```python
from build123d import *

# Parameters (mm, degrees)
SKETCH_1_R          = 70
EXTRUDE_1_DEPTH     = 525
SKETCH_2_OUTSIDE_W  = 254.218
SKETCH_2_OUTSIDE_H  = 254.218
SKETCH_2_OUTSIDE_R  = 45
CUT_EXTRUDE_2_DEPTH = 285
CUT_EXTRUDE_START   = -20
SKETCH_3_OUTSIDE_W  = 254.218
SKETCH_3_OUTSIDE_H  = 254.218
SKETCH_3_OUTSIDE_R  = 60
CUT_EXTRUDE_3_DEPTH = 282.703496831
SKETCH_4_OUTSIDE_W  = 254.218
SKETCH_4_OUTSIDE_H  = 254.218
SKETCH_4_OUTSIDE_R  = 37.5
CUT_EXTRUDE_4_DEPTH = 232.5
SKETCH_5_OUTSIDE_W  = 254.218
SKETCH_5_OUTSIDE_H  = 254.218
SKETCH_5_OUTSIDE_R  = 37.5
CUT_EXTRUDE_5_DEPTH = 120
CUT_EXTRUDE_START_2 = 50
CUT_EXTRUDE_6_DEPTH = 485.251813287
SKETCH_8_OUTSIDE_W  = 254.218
SKETCH_8_OUTSIDE_H  = 254.218
SKETCH_8_OUTSIDE_R  = 34
CUT_EXTRUDE_1_DEPTH = 130
CUT_EXTRUDE_START_3 = 30.5
CUT_EXTRUDE_7_DEPTH = 504.751813287
FILLET_1_R          = 5


with BuildPart() as part:
    # 草图1 → 拉伸1 (new body)
    with BuildSketch(Plane(origin=(0, 0, 0), x_dir=(0, 0, -1), z_dir=(1, 0, 0))):
        Circle(SKETCH_1_R)
    extrude(amount=EXTRUDE_1_DEPTH)

    # 草图2 outside → 拉伸2 (cut)
    with BuildSketch(Plane(origin=(525, 0, 0), x_dir=(0, 0, -1), z_dir=(1, 0, 0))):
        Rectangle(SKETCH_2_OUTSIDE_W, SKETCH_2_OUTSIDE_H)
        Circle(SKETCH_2_OUTSIDE_R, mode=Mode.SUBTRACT)
    extrude(amount=-CUT_EXTRUDE_2_DEPTH, mode=Mode.SUBTRACT)

    # 草图3 outside → 拉伸3 (cut, through all)
    with BuildSketch(Plane(origin=(240, 0, 0), x_dir=(0, 0, -1), z_dir=(1, 0, 0)).offset(CUT_EXTRUDE_START)):
        Rectangle(SKETCH_3_OUTSIDE_W, SKETCH_3_OUTSIDE_H)
        Circle(SKETCH_3_OUTSIDE_R, mode=Mode.SUBTRACT)
    extrude(amount=-CUT_EXTRUDE_3_DEPTH, mode=Mode.SUBTRACT)

    # 草图4 outside → 拉伸4 (cut)
    with BuildSketch(Plane(origin=(525, 0, 0), x_dir=(0, 0, -1), z_dir=(1, 0, 0))):
        Rectangle(SKETCH_4_OUTSIDE_W, SKETCH_4_OUTSIDE_H)
        Circle(SKETCH_4_OUTSIDE_R, mode=Mode.SUBTRACT)
    extrude(amount=-CUT_EXTRUDE_4_DEPTH, mode=Mode.SUBTRACT)

    # 草图5 outside → 拉伸5 (cut)
    with BuildSketch(Plane.ZY):
        Rectangle(SKETCH_5_OUTSIDE_W, SKETCH_5_OUTSIDE_H)
        with Locations(Location((0, 0, 0), (0, 0, 180))):
            Circle(SKETCH_5_OUTSIDE_R, mode=Mode.SUBTRACT)
    extrude(amount=-CUT_EXTRUDE_5_DEPTH, mode=Mode.SUBTRACT)

    # 草图6 → 拉伸6 (cut, through all)
    with BuildSketch(Plane.XY.offset(CUT_EXTRUDE_START_2)):
        with BuildLine():
            Line((146, 16), (189, 16))
            ThreePointArc((189, 16), (205, 0), (189, -16))
            Line((189, -16), (146, -16))
            ThreePointArc((146, -16), (130, 0), (146, 16))
        make_face()
    extrude(amount=CUT_EXTRUDE_6_DEPTH, mode=Mode.SUBTRACT)

    # 草图8 outside → 切除-拉伸1 (cut)
    with BuildSketch(Plane(origin=(525, 0, 0), x_dir=(0, 0, -1), z_dir=(1, 0, 0))):
        Rectangle(SKETCH_8_OUTSIDE_W, SKETCH_8_OUTSIDE_H)
        Circle(SKETCH_8_OUTSIDE_R, mode=Mode.SUBTRACT)
    extrude(amount=-CUT_EXTRUDE_1_DEPTH, mode=Mode.SUBTRACT)

    # 草图7 → 拉伸7 (cut, through all)
    with BuildSketch(Plane.XY.offset(CUT_EXTRUDE_START_3)):
        with BuildLine():
            Line((421, 11), (499, 11))
            ThreePointArc((499, 11), (510, 0), (499, -11))
            Line((499, -11), (421, -11))
            ThreePointArc((421, -11), (410, 0), (421, 11))
        make_face()
    extrude(amount=CUT_EXTRUDE_7_DEPTH, mode=Mode.SUBTRACT)

    # 圆角1
    fillet_1_edges = [part.edges().sort_by_distance(p)[0] for p in [
        (292.5, 0, 37.5),
        (120, 0, 37.5),
    ]]
    fillet(fillet_1_edges, radius=FILLET_1_R)


solid = part.part
```
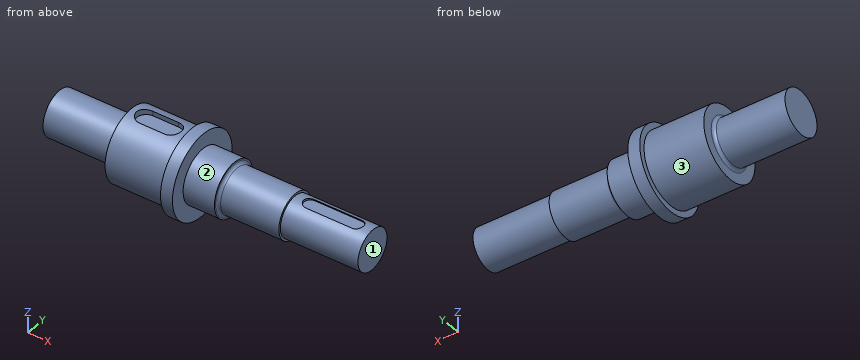
Build history of the part. All positions in model axes, mm. Face numbers are marked on the shaded views. A direction names the side the tool comes from. Give positions to 0.01 mm unless a question says otherwise; leave off trailing zeros. Loops run counter-clockwise (first coordinate to the right, second up) from the corner with the lowest first, then second, coordinate; pieces in that order, holes last.
1) Drop flat-ended pins along their axis: P1, Ø8, axis at x = 211.5, z = 50.5, coming from the +Y side; P2, Ø1, axis at y = 48.5, z = -36, coming from the -X side; P3, Ø10, axis at x = 96, z = -44, coming from the +Y side; P4, Ø1.8, axis at x = 462, z = 31, coming from the +Y side. Give the stop position or say it passes through.
Values follow:
P1: stops at y = 37.92
P2: stops at x = 120
P3: passes through
P4: stops at y = 15.81
2) Band-saw the part on C-C on x = 161. List the corners of the cut face in (y, z).
Values follow:
outline: (-16, 50) - (-16, 57.83) arc R60 ccw (long way) to (16, 57.83) - (16, 50) - close
3) 3-axis set-ups, long thin cutter, end or side, ignore diameter. For the marked faces 1, 2 and 3: which of +Z, -Z, +X, -X, +Y, -Y reach the whole face in a straight line?
Values follow:
face 1: +Z, -Z, +X, +Y, -Y
face 2: +X
face 3: -X
4) Band-saw the part on D-D on x = 310. List the corners of the cut face in (y, z).
Values follow:
outline: circle Ø75 at (0, 0)
5) Band-saw the part on B-B on x = 438.5. List the corners of the cut face in (y, z), then the cut area to 3 significant figures.
Values follow:
outline: (-11, 30.5) - (-11, 32.17) arc R34 ccw (long way) to (11, 32.17) - (11, 30.5) - close
area: 3,570 mm2
6) Band-saw the part on A-A on z = 0. List the corners of the cut face in (x, y), then the cut area to 3 significant figures.
Values follow:
outline: (0, -37.5) - (115, -37.5) arc R5 cw to (120, -42.5) - (120, -60) - (220, -60) - (220, -70) - (240, -70) - (240, -45) - (292.5, -45) - (292.5, -42.5) arc R5 cw to (297.5, -37.5) - (395, -37.5) - (395, -34) - (525, -34) - (525, 34) - (395, 34) - (395, 37.5) - (297.5, 37.5) arc R5 cw to (292.5, 42.5) - (292.5, 45) - (240, 45) - (240, 70) - (220, 70) - (220, 60) - (120, 60) - (120, 42.5) arc R5 cw to (115, 37.5) - (0, 37.5) - close
area: 45,100 mm2
7) Probe line 1 along X through (y, z) = (-28.5, -32.5); line 2 along X through (y, z) = (-37, 19); line 3 along Y through (x, z) = (402.5, -2). List the from-to ranges inside material, lowest first.
Values follow:
line 1: x = 120 to 292.5
line 2: x = 119.92 to 292.58
line 3: y = -33.94 to 33.94
